The model under review builds one solid part; all positions refer to its coordinate system, in mm. A direction names the side the tool comes from. Round coordinates to 2 decimals unless told otherwise and drop trailing zeros. Write each loop counter-clockwise with the first axis right and the second up, starting at its lowest first coordinate (ties: lowest second). Pieces come first, ordered by that corner, then holes. Notation, with made-up numbers: (-5, 46.5) -> (37, 46.5) arc R21 ccw to (37, 66.5) -> close; hole circle Ø5 at (69, -6). An arc over 180 degrees is marked (long way). Answer as a JSON object with one key per item and string values. Group by question number.
1) We need section D-D, the plane x = 5.75. Write out the cut boundary in (y, z).
2) We need section B-B, the plane z = 1.25. Write out the cut boundary in (x, y).
3) We need section C-C, the plane x = 9. Write out the cut boundary in (y, z).
4) Mouldability with a two-part tool opening along X and no side actions: class faces 4 (the flat face through (3, 19, 2)), 5 (the cylindrical face through (10.54, 7.56, 2.96)), 6 (the cylindrical face through (11.75, 18.61, 0.99)) as pulls with the +X half, pulls with the -X half, needs draft (parallel to the pull), parting line crosses it, or undercut.
5) Machinability: for faces 1 (the flat face through (10, 0, 3)), 2 (the flat face through (18, 13.5, 1)), 3 (the flat face through (2, 13.5, 1)), which of the approach directions +Z, -Z, +X, -X, +Y, -Y give a long, thin tool a straight path to every point of the face, cutting with its end or side? Answer none if there is none.
6) To check wall thickness, follow probe 1 along Y at (x, z) = (10, 3.1); probe 2 along Y at (x, z) = (1, 1.8); probe 3 along Y at (x, z) = (9, 2.1). State the ranges of each line that lie inside material, in increasing order. Write a range as [from, to].
7) We need section A-A, the plane y = 35. Write out the cut boundary in (x, z).
8) Insertion check: pin 1 Ø2.5 at (x, y) = (15.5, 17.5) entering from -Z; pin 2 Ø4 at (x, y) = (10, 35) entering from -Z. Each pin has a flat end and moves straight along its axis. Give the tip position at first contact, or say it passes through.
from build123d import *

# Parameters (mm, degrees)
ESBO_O1_W                = 20
ESBO_O1_H                = 50
RESSALTO_EXTRUS_O1_DEPTH = 6
ESBO_O2_R                = 2.5
CORTE_EXTRUS_O1_DEPTH    = 10
ESBO_O3_R                = 5
CORTE_EXTRUS_O2_DEPTH    = 2
ESBO_O4_W                = 3.25
ESBO_O4_H                = 10
CORTE_EXTRUS_O3_DEPTH    = 2
ESBO_O5_R                = 2.5
RESSALTO_EXTRUS_O2_DEPTH = 4


with BuildPart() as part:
    # Esboço1 → Ressalto-extrusão1 (new body)
    with BuildSketch(Plane.XY):
        with Locations((10, 25)):
            Rectangle(ESBO_O1_W, ESBO_O1_H)
    extrude(amount=RESSALTO_EXTRUS_O1_DEPTH)

    # Esboço2 → Corte-extrusão1 (cut)
    with BuildSketch(Plane(origin=(0, 0, 0), x_dir=(-1, 0, 0), z_dir=(0, 0, -1))):
        with Locations((-10, 35)):
            Circle(ESBO_O2_R)
        with Locations((-3.25, 18.5)):
            Circle(ESBO_O2_R)
        with Locations((-10, 10)):
            Circle(ESBO_O2_R)
    extrude(amount=-CORTE_EXTRUS_O1_DEPTH, mode=Mode.SUBTRACT)

    # Esboço3 → Corte-extrusão2 (cut)
    with BuildSketch(Plane.XY):
        with Locations((3.25, 18.5)):
            Circle(ESBO_O3_R)
        with Locations((16.75, 18.5)):
            Circle(ESBO_O3_R)
    extrude(amount=CORTE_EXTRUS_O2_DEPTH, mode=Mode.SUBTRACT)

    # Esboço4 → Corte-extrusão3 (cut)
    with BuildSketch(Plane(origin=(0, 0, 0), x_dir=(-1, 0, 0), z_dir=(0, 0, -1))):
        with Locations((-1.625, 18.5)):
            Rectangle(ESBO_O4_W, ESBO_O4_H)
        with Locations((-18.375, 18.5)):
            Rectangle(ESBO_O4_W, ESBO_O4_H)
    extrude(amount=-CORTE_EXTRUS_O3_DEPTH, mode=Mode.SUBTRACT)

    # Esboço5 → Ressalto-extrusão2 (add)
    with BuildSketch(Plane.XY.offset(6)):
        with Locations((3.25, 18.5)):
            Circle(ESBO_O5_R)
    extrude(amount=-RESSALTO_EXTRUS_O2_DEPTH)


solid = part.part
Here are the results:
{
 "1": {"outline": "(0, 0) -> (14.17, 0) -> (14.17, 2) -> (22.83, 2) -> (22.83, 0) -> (50, 0) -> (50, 6) -> (0, 6) -> close"},
 "2": {"outline": "(0, 0) -> (20, 0) -> (20, 13.5) -> (16.75, 13.5) arc R5 cw to (16.75, 23.5) -> (20, 23.5) -> (20, 50) -> (0, 50) -> (0, 23.5) -> (3.25, 23.5) arc R5 cw to (3.25, 13.5) -> (0, 13.5) -> close; hole circle Ø5 at (10, 10); hole circle Ø5 at (10, 35)"},
 "3": {"outline": "(0, 0) -> (7.71, 0) -> (7.71, 6) -> (0, 6) -> close; (12.29, 0) -> (32.71, 0) -> (32.71, 6) -> (12.29, 6) -> close; (37.29, 0) -> (50, 0) -> (50, 6) -> (37.29, 6) -> close"},
 "4": {"face 4": "needs draft", "face 5": "undercut", "face 6": "pulls with the +X half"},
 "5": {"face 1": "+Z, -Z, +X, -X, -Y", "face 2": "-Z, +X", "face 3": "-Z, -X"},
 "6": {"probe 1": "y = [0, 7.5], [12.5, 32.5], [37.5, 50]", "probe 2": "y = [0, 13.5], [23.5, 50]", "probe 3": "y = [0, 7.71], [12.29, 32.71], [37.29, 50]"},
 "7": {"outline": "(0, 0) -> (7.5, 0) -> (7.5, 6) -> (0, 6) -> close; (12.5, 0) -> (20, 0) -> (20, 6) -> (12.5, 6) -> close"},
 "8": {"pin 1": "stops at z = 2", "pin 2": "passes through"}
}
